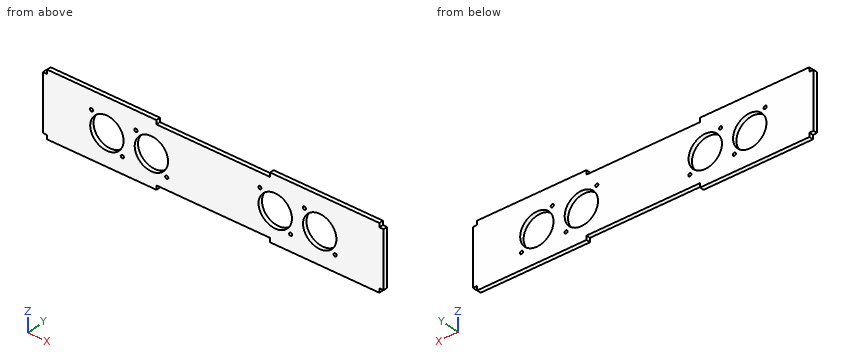
from build123d import *

# Parameters (mm, degrees)
SKETCH2_W                 = 490
SKETCH2_H                 = 94.85
BOSS_EXTRUDE1_DEPTH       = 6
SKETCH4_W                 = 6
SKETCH4_H                 = 6
CUT_EXTRUDE2_DEPTH        = 500.131768674
SKETCH5_W                 = 163.333333334
SKETCH5_H                 = 6
CUT_EXTRUDE3_DEPTH        = 500.131768674
M4_CLEARANCE_SLOT1_D      = 4.5
M4_CLEARANCE_SLOT1_DEPTH  = 18
M4_CLEARANCE_SLOT1_TIP    = 1.351936393
M45_CLEARANCE_SLOT1_D     = 48
M45_CLEARANCE_SLOT1_DEPTH = 18
M45_CLEARANCE_SLOT1_TIP   = 14.420654857


with BuildPart() as part:
    # Sketch2 → Boss-Extrude1 (new body)
    with BuildSketch(Plane(origin=(0, 0, 0), x_dir=(1, 0, 0), z_dir=(0, 1, 0))):
        with Locations((245, 47.425)):
            Rectangle(SKETCH2_W, SKETCH2_H)
    extrude(amount=BOSS_EXTRUDE1_DEPTH)

    # Sketch4 → Cut-Extrude2 (cut, through all)
    with BuildSketch(Plane(origin=(0, 6, 0), x_dir=(1, 0, 0), z_dir=(0, 1, 0))):
        with Locations((487, 3)):
            Rectangle(SKETCH4_W, SKETCH4_H)
        with Locations((487, 91.85)):
            Rectangle(SKETCH4_W, SKETCH4_H)
        with Locations((3, 91.85)):
            Rectangle(SKETCH4_W, SKETCH4_H)
        with Locations((3, 3)):
            Rectangle(SKETCH4_W, SKETCH4_H)
    extrude(amount=-CUT_EXTRUDE2_DEPTH, mode=Mode.SUBTRACT)

    # Sketch5 → Cut-Extrude3 (cut, through all)
    with BuildSketch(Plane(origin=(0, 6, 0), x_dir=(1, 0, 0), z_dir=(0, 1, 0))):
        with Locations((245, 91.85)):
            Rectangle(SKETCH5_W, SKETCH5_H)
        with Locations((245, 3)):
            Rectangle(SKETCH5_W, SKETCH5_H)
    extrude(amount=-CUT_EXTRUDE3_DEPTH, mode=Mode.SUBTRACT)

    # M4 Clearance Slot1
    with Locations(Plane(origin=(0, 6, 0), x_dir=(1, 0, 0), z_dir=(0, 1, 0))):
        with Locations((375.95208337, 26.806250977), (420.25208337, 71.106250977), (356.25208337, 71.106250977), (311.95208337, 26.806250977), (178.04791663, 71.106250977), (133.74791663, 26.806250977), (114.04791663, 71.106250977), (69.74791663, 26.806250977)):
            Hole(M4_CLEARANCE_SLOT1_D / 2, depth=M4_CLEARANCE_SLOT1_DEPTH)
            with Locations((0, 0, -(M4_CLEARANCE_SLOT1_DEPTH + M4_CLEARANCE_SLOT1_TIP / 2))):  # 118° drill point
                Cone(0, M4_CLEARANCE_SLOT1_D / 2, M4_CLEARANCE_SLOT1_TIP, mode=Mode.SUBTRACT)

    # M45 Clearance Slot1
    with Locations(Plane(origin=(0, 6, 0), x_dir=(1, 0, 0), z_dir=(0, 1, 0))):
        with Locations((91.89791663, 48.956250977), (155.89791663, 48.956250977), (334.10208337, 48.956250977), (398.10208337, 48.956250977)):
            Hole(M45_CLEARANCE_SLOT1_D / 2, depth=M45_CLEARANCE_SLOT1_DEPTH)
            with Locations((0, 0, -(M45_CLEARANCE_SLOT1_DEPTH + M45_CLEARANCE_SLOT1_TIP / 2))):  # 118° drill point
                Cone(0, M45_CLEARANCE_SLOT1_D / 2, M45_CLEARANCE_SLOT1_TIP, mode=Mode.SUBTRACT)


solid = part.part
Design review of the part built by this model. Coordinates are the model's own, in mm. Coordinates: 2 decimals unless noted, no trailing zeros. Order: outer loops, then holes, each group sorted by start corner. A loop starts at its lowest first (then second) coordinate and runs counter-clockwise, first axis right, second up.
Item 1: Take a section at B-B, the plane y = 5.1. Count the separate pieces of the cut face and the enclosed holes in it, then the cut area to 3 significant figures.
Item 2: For line 1 (X direction, y = 0.4, z = -50); line 2 (X direction, y = 0.75, z = -37); line 3 (Z direction, x = 333, y = 0.75), list the stretches that pass through material, from the lowest coordinate up.
Item 3: Take a section at A-A, the plane z = -41. Write out the cut boundary in (x, y), then the cut area to 3 significant figures.
Item 4: Take a section at C-C, the plane x = 192.5. Write out the cut boundary in (y, z).
Item 5: For pin 1 Ø1.8 at (y, z) = (1.5, -1.5) entering from +X; pin 2 Ø1.5 at (y, z) = (2, -19.5) entering from -X; pin 3 Ø1 at (x, y) = (211.5, 3) entering from -Z; pin 4 Ø1.8 at (x, y) = (4, 3.5) entering from +Z, all flat-tipped, find the tip position at first contact; note any pin that passes through.
Item 6: Take a section at D-D, the plane z = -64.5. Write out the cut boundary in (x, y).
The answers:
1. separate pieces: 1
1. enclosed holes: 12
1. area: 37,000 mm2
2. line 1: x = 0 to 67.92, 115.88 to 131.92, 179.88 to 310.12, 358.08 to 374.12, 422.08 to 490
2. line 2: x = 0 to 71.09, 112.71 to 135.09, 176.71 to 313.29, 354.91 to 377.29, 418.91 to 490
2. line 3: z = -94.85 to -72.93, -24.98 to 0
3. outline: (0, 0) - (69.26, 0) - (69.26, 6) - (0, 6) - close; (114.54, 0) - (133.26, 0) - (133.26, 6) - (114.54, 6) - close; (178.54, 0) - (311.46, 0) - (311.46, 6) - (178.54, 6) - close; (356.74, 0) - (375.46, 0) - (375.46, 6) - (356.74, 6) - close; (420.74, 0) - (490, 0) - (490, 6) - (420.74, 6) - close
3. area: 1,850 mm2
4. outline: (0, -88.85) - (6, -88.85) - (6, -6) - (0, -6) - close
5. pin 1: stops at x = 484
5. pin 2: stops at x = 0
5. pin 3: stops at z = -88.85
5. pin 4: stops at z = -6
6. outline: (0, 0) - (73.61, 0) - (73.61, 6) - (0, 6) - close; (110.18, 0) - (137.61, 0) - (137.61, 6) - (110.18, 6) - close; (174.18, 0) - (315.82, 0) - (315.82, 6) - (174.18, 6) - close; (352.39, 0) - (379.82, 0) - (379.82, 6) - (352.39, 6) - close; (416.39, 0) - (490, 0) - (490, 6) - (416.39, 6) - close
